from build123d import *

# Parameters (mm, degrees)
F0_W     = 94
F0_H     = 45
F1_DEPTH = 19
F2_W     = 31
F2_H     = 27
F3_DEPTH = 38.001
F4_R     = 10
F5_DEPTH = 45.001
F6_W     = 8
F6_H     = 32
F7_DEPTH = 16
F9_DEPTH = 9


# Not quite as in the source:
# - a pattern or mirror of a feature is missing from the dataset's text; its kind, count and spacing are read off the source's solid


with BuildPart() as f1:
    # F0 (on Right) → F1 (new body, symmetric)
    with BuildSketch(Plane.YZ):
        Rectangle(F0_W, F0_H)
    extrude(amount=F1_DEPTH, both=True)

    # F2 (on face) → F3 (cut, through all)
    with BuildSketch(Plane.YZ.offset(19)):
        with Locations((-31.5, 9)):
            Rectangle(F2_W, F2_H)
    f3 = extrude(amount=-F3_DEPTH, mode=Mode.SUBTRACT)

    # F3_copies: F3 across plane
    add(f3.mirror(Plane.ZX), mode=Mode.SUBTRACT)

    # F4 (on face) → F5 (cut, through all)
    with BuildSketch(Plane.XY.offset(22.5)):
        Circle(F4_R)
    extrude(amount=-F5_DEPTH, mode=Mode.SUBTRACT)

    # F6 (on face) → F7 (cut)
    with BuildSketch(Plane.XY.offset(22.5)):
        Rectangle(F6_W, F6_H)
    extrude(amount=-F7_DEPTH, mode=Mode.SUBTRACT)

    # F8 (on Right) → F9 (cut, symmetric)
    with BuildSketch(Plane.YZ):
        Polygon((-25, -4.5), (-47, -4.5), (-47, -22.5), align=None)
    f9 = extrude(amount=F9_DEPTH, both=True, mode=Mode.SUBTRACT)

    # F9_copies: F9 across plane
    add(f9.mirror(Plane.ZX), mode=Mode.SUBTRACT)


solid = f1.part
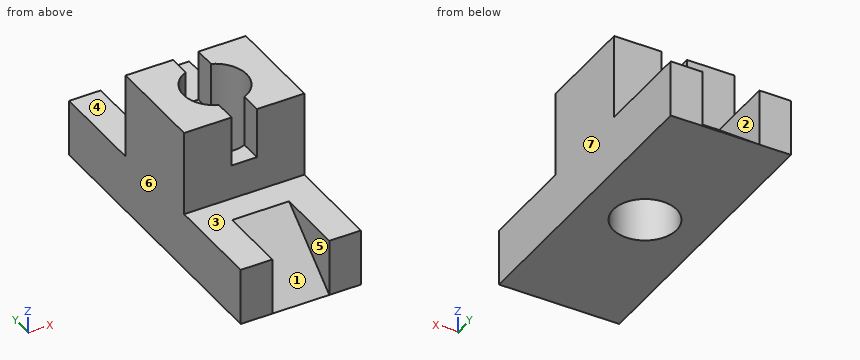
Can you work these out from the model? Positions are in its coordinate system, mm. Face numbers are marked on the shaded views. A direction names the side the tool comes from. Coordinates: 2 decimals unless noted, no trailing zeros. Loops run counter-clockwise (first coordinate to the right, second up) from the corner with the lowest first, then second, coordinate; pieces in that order, holes last. Notation, with made-up numbers: M 71.25,-26.5 L 123.25,-26.5 A23 cw 123.25,-13.5 Z; hole C 74,26.25 d9. An arc over 180 degrees is marked long. Return JSON: item names as keys, results as strings. Group by question number.
Item 1: Thinking about a two-plate mould opening in X: for the marked faces 5, 6 and 7, which applies, released by +X, released by -X, zero draft, split by the parting line, or undercut?
Item 2: On a 3-axis mill with a long thin cutter (end or side, diameter ignored), from which of +Z, -Z, +X, -X, +Y, -Y can I reach the whole of each face in a straight line? I mean the marked faces 1, 2, 3 and 4. Say none if no direction works.
Item 3: Imagine slicing it at B-B (z = 9.5). Please give me the cut outline in (x, y).
Item 4: Imagine slicing it at D-D (y = 12.5). Please give me the cut outline in (x, z).
Item 5: Imagine slicing it at A-A (y = 0). Please give me the cut outline in (x, z).
Item 6: Imagine slicing it at C-C (x = 0). Please give me the cut outline in (y, z).
Item 7: I'm going to push flat-ended pins straight in: pin 1 Ø5.5 at (x, y) = (-0.5, 11) entering from +Z; pin 2 Ø1.5 at (x, z) = (-3.5, -7) entering from -Y; pin 3 Ø1 at (x, y) = (-9.5, 28.5) entering from +Z. Where does each tip first touch, or does it pass through?
Item 8: If I drill on L1, parallel to Y at x = 0, z = 2.5; L2, parallel to Z at x = -8, y = 21; L3, parallel to Y at x = 15.5, z = 9.5, over which ranges is the centre line in solid material (lowest first)? Write a range as from..to.
Verdict:
{
 "1": {"face 5": "undercut", "face 6": "released by -X", "face 7": "released by +X"},
 "2": {"face 1": "+Z, -Y", "face 2": "+Z, +Y", "face 3": "+Z, +X, -X, -Y", "face 4": "+Z, +X, -X, +Y"},
 "3": {"outline": "M -19,-16 L -4,-16 L -4,-9.17 A10 cw -4,9.17 L -4,16 L -19,16 Z; M 4,-16 L 19,-16 L 19,16 L 4,16 L 4,9.17 A10 cw 4,-9.17 Z"},
 "4": {"outline": "M -19,-22.5 L 19,-22.5 L 19,22.5 L 4,22.5 L 4,6.5 L -4,6.5 L -4,22.5 L -19,22.5 Z"},
 "5": {"outline": "M -19,-22.5 L -10,-22.5 L -10,22.5 L -19,22.5 Z; M 10,-22.5 L 19,-22.5 L 19,22.5 L 10,22.5 Z"},
 "6": {"outline": "M -47,-22.5 L -10,-22.5 L -10,6.5 L -16,6.5 L -16,-4.5 L -25,-4.5 Z; M 10,-22.5 L 47,-22.5 L 25,-4.5 L 16,-4.5 L 16,6.5 L 10,6.5 Z"},
 "7": {"pin 1": "stops at z = 6.5", "pin 2": "stops at y = -28.97", "pin 3": "stops at z = -4.5"},
 "8": {"L1": "y = -16..-10, 10..16", "L2": "z = -22.5..-4.5", "L3": "y = -16..16"}
}
